Verification items for the finished model (mm, model axes). A direction names the side the tool comes from. Coordinates: 2 decimals unless noted, no trailing zeros. Write each loop counter-clockwise with the first axis right and the second up, starting at its lowest first coordinate (ties: lowest second). Pieces come first, ordered by that corner, then holes. Notation, with made-up numbers: (15.25, 52.25) -> (68.25, 52.25) arc R22 ccw to (68.25, 63.25) -> close; hole circle Ø3 at (47, 72.25). An arc over 180 degrees is marked (long way). Answer in a Markdown table with one row per item.
```python
from build123d import *

# Parameters (mm, degrees)
SKETCH7_W           = 50
SKETCH7_H           = 15
SKETCH7_R           = 2.25
SKETCH7_R_2         = 2.75
SKETCH7_W_2         = 19
SKETCH7_H_2         = 29.5
BOSS_EXTRUDE3_DEPTH = 6
SKETCH8_R           = 3.75
CUT_EXTRUDE4_DEPTH  = 2.1


with BuildPart() as part:
    # Sketch7 → Boss-Extrude3 (new body)
    # profile 1 of 2: a face of its own
    with BuildSketch(Plane.XY):
        Rectangle(SKETCH7_W, SKETCH7_H)
        Circle(SKETCH7_R, mode=Mode.SUBTRACT)
        with Locations((-16, 0)):
            Circle(SKETCH7_R_2, mode=Mode.SUBTRACT)
        with Locations((16, 0)):
            Circle(SKETCH7_R_2, mode=Mode.SUBTRACT)
    # profile 2 of 2: a face of its own
    with BuildSketch(Plane.XY):
        with Locations((0, -22.25)):
            Rectangle(SKETCH7_W_2, SKETCH7_H_2)
        with Locations((0, -30)):
            Circle(SKETCH7_R, mode=Mode.SUBTRACT)
    extrude(amount=BOSS_EXTRUDE3_DEPTH)

    # Sketch8 → Cut-Extrude4 (cut)
    with BuildSketch(Plane.XY.offset(6)):
        Circle(SKETCH8_R)
        with Locations((0, -30)):
            Circle(SKETCH8_R)
    extrude(amount=-CUT_EXTRUDE4_DEPTH, mode=Mode.SUBTRACT)


solid = part.part
```
1. Sectioned sample at A-A, the plane y = 0. Record the cut outline in (x, z).
Findings below:
| item | result |
|---|---|
| outline | (-25, 0) -> (-18.75, 0) -> (-18.75, 6) -> (-25, 6) -> close; (-13.25, 0) -> (-2.25, 0) -> (-2.25, 3.9) -> (-3.75, 3.9) -> (-3.75, 6) -> (-13.25, 6) -> close; (2.25, 0) -> (13.25, 0) -> (13.25, 6) -> (3.75, 6) -> (3.75, 3.9) -> (2.25, 3.9) -> close; (18.75, 0) -> (25, 0) -> (25, 6) -> (18.75, 6) -> close |
2. Sectioned sample at B-B, the plane x = -16. Record the cut outline in (y, z).
Findings below:
| item | result |
|---|---|
| outline | (-7.5, 0) -> (-2.75, 0) -> (-2.75, 6) -> (-7.5, 6) -> close; (2.75, 0) -> (7.5, 0) -> (7.5, 6) -> (2.75, 6) -> close |
3. Release check for a two-part mould opening along X. For faces 1 (the face through (25, 0, 3)), 2 (the face through (2, -32, 3.9)), 3 (the face through (17, -7.5, 3)) record: released by +X, released by -X, zero draft, split by the parting line, or undercut.
Findings below:
| item | result |
|---|---|
| face 1 | released by +X |
| face 2 | undercut |
| face 3 | zero draft |
4. Sectioned sample at D-D, the plane x = 0. Record the cut outline in (y, z), and give its area (3 significant figures).
Findings below:
| item | result |
|---|---|
| outline | (-37, 0) -> (-32.25, 0) -> (-32.25, 3.9) -> (-33.75, 3.9) -> (-33.75, 6) -> (-37, 6) -> close; (-27.75, 0) -> (-2.25, 0) -> (-2.25, 3.9) -> (-3.75, 3.9) -> (-3.75, 6) -> (-26.25, 6) -> (-26.25, 3.9) -> (-27.75, 3.9) -> close; (2.25, 0) -> (7.5, 0) -> (7.5, 6) -> (3.75, 6) -> (3.75, 3.9) -> (2.25, 3.9) -> close |
| area | 200 mm² |
5. Go/stop test with flat-tipped pins: pin 1 (3 mm diameter, centred on y = -21.5, z = 3.5, fed in from -X); pin 2 (1.8 mm diameter, centred on y = -17.5, z = 3, fed in from +X); pin 3 (1.5 mm diameter, centred on x = -10.5, z = 4.5, fed in from -Y). Record where each tip stops, or that it passes through.
Findings below:
| item | result |
|---|---|
| pin 1 | stops at x = -9.5 |
| pin 2 | stops at x = 9.5 |
| pin 3 | stops at y = -7.5 |
6. Material ranges on probe 1 along Y at (x, z) = (0, 1.4); probe 2 along Y at (x, z) = (0, 5.35); probe 3 along Y at (x, z) = (-16, 4.55), recorded low to high. Write a range as from..to.
Findings below:
| item | result |
|---|---|
| probe 1 | y = -37..-32.25, -27.75..-2.25, 2.25..7.5 |
| probe 2 | y = -37..-33.75, -26.25..-3.75, 3.75..7.5 |
| probe 3 | y = -7.5..-2.75, 2.75..7.5 |
7. Access from +Z, -Z, +X, -X, +Y, -Y to the whole of each face (thin tool, end or side, straight path). Record for faces 4 (the face through (0, -37, 3)), 5 (the face through (2, -2, 3.9)), 6 (the face through (0, -9, 0)), 7 (the face through (9.5, -22, 3)), 8 (the face through (-9.5, -22, 3)).
Findings below:
| item | result |
|---|---|
| face 4 | +Z, -Z, +X, -X, -Y |
| face 5 | +Z |
| face 6 | -Z, +X, -X, +Y, -Y |
| face 7 | +Z, -Z, +X, -Y |
| face 8 | +Z, -Z, -X, -Y |
8. Sectioned sample at C-C, the plane z = 0.85. Record the cut outline in (x, y).
Findings below:
| item | result |
|---|---|
| outline | (-25, -7.5) -> (-9.5, -7.5) -> (-9.5, -37) -> (9.5, -37) -> (9.5, -7.5) -> (25, -7.5) -> (25, 7.5) -> (-25, 7.5) -> close; hole circle Ø5.5 at (-16, 0); hole circle Ø4.5 at (0, -30); hole circle Ø4.5 at (0, 0); hole circle Ø5.5 at (16, 0) |
